Part model, mm, in its own coordinate system. Face numbers are marked on the shaded views. A direction names the side the tool comes from. Round coordinates to 2 decimals unless told otherwise and drop trailing zeros. Loops run counter-clockwise (first coordinate to the right, second up) from the corner with the lowest first, then second, coordinate; pieces in that order, holes last. Notation, with made-up numbers: (-3.75, 13.5) -> (38.25, 13.5) arc R21 cw to (38.25, 47.5) -> close; hole circle Ø2 at (55, 43). An arc over 180 degrees is marked (long way). Answer as CSV lines item,"result".
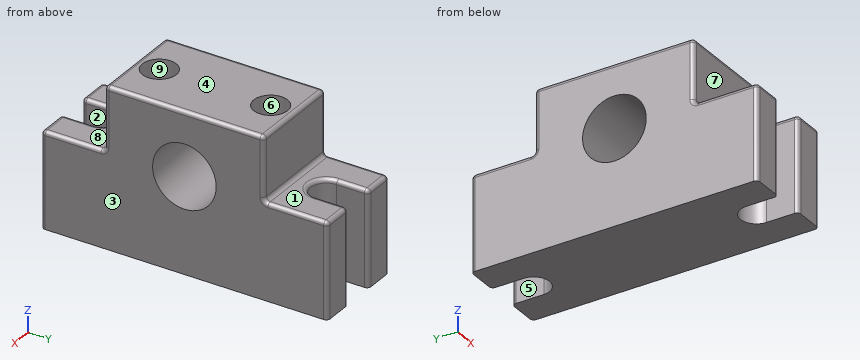
from build123d import *

# Parameters (mm, degrees)
F0_W     = 19.05
F0_H     = 6.35
F0_H_2   = 15.875
F0_R     = 3.571875
F0_H_3   = 9.525
F1_DEPTH = 19.05
F2_DEPTH = 31.75
F4_D     = 12.7
F6_D     = 6.7564
F6_DEPTH = 12.7
F6_TIP   = 2.0298273432
F7_R     = 0.79375


with BuildPart() as f1:
    # F0 (on Top) → F1 (new body)
    with BuildSketch(Plane.XY):
        with Locations((0, 3.175)):
            Rectangle(F0_W, F0_H)
        with BuildLine():
            Line((9.525, -28.575), (9.525, -15.875))
            Line((9.525, -15.875), (-9.525, -15.875))
            Line((-9.525, -15.875), (-9.525, -28.575))
            Line((-9.525, -28.575), (-3.175, -28.575))
            Line((-3.175, -28.575), (-3.175, -22.225))
            ThreePointArc((-3.175, -22.225), (0, -19.05), (3.175, -22.225))
            Line((3.175, -22.225), (3.175, -28.575))
            Line((3.175, -28.575), (9.525, -28.575))
        make_face()
        with Locations((0, -7.9375)):
            Rectangle(F0_W, F0_H_2)
        with Locations((0, -11.1125)):
            Circle(F0_R, mode=Mode.SUBTRACT)
        with Locations((0, 11.1125)):
            Rectangle(F0_W, F0_H_3)
        with Locations((0, 11.1125)):
            Circle(F0_R, mode=Mode.SUBTRACT)
        with BuildLine():
            Line((9.525, 15.875), (9.525, 28.575))
            Line((9.525, 28.575), (3.175, 28.575))
            Line((3.175, 28.575), (3.175, 22.225))
            ThreePointArc((3.175, 22.225), (0, 19.05), (-3.175, 22.225))
            Line((-3.175, 22.225), (-3.175, 28.575))
            Line((-3.175, 28.575), (-9.525, 28.575))
            Line((-9.525, 28.575), (-9.525, 15.875))
            Line((-9.525, 15.875), (9.525, 15.875))
        make_face()
        with Locations((0, 11.1125)):
            Circle(F0_R)
        with Locations((0, -11.1125)):
            Circle(F0_R)
    extrude(amount=F1_DEPTH)

    # F0 (on Top) → F2 (join)
    with BuildSketch(Plane.XY):
        with Locations((0, 3.175)):
            Rectangle(F0_W, F0_H)
        with Locations((0, -7.9375)):
            Rectangle(F0_W, F0_H_2)
        with Locations((0, -11.1125)):
            Circle(F0_R, mode=Mode.SUBTRACT)
        with Locations((0, 11.1125)):
            Rectangle(F0_W, F0_H_3)
        with Locations((0, 11.1125)):
            Circle(F0_R, mode=Mode.SUBTRACT)
        with Locations((0, -11.1125)):
            Circle(F0_R)
        with Locations((0, 11.1125)):
            Circle(F0_R)
    extrude(amount=F2_DEPTH)

    # F4 (through all)
    with Locations(Plane.YZ.offset(9.525)):
        with Locations((0, 19.05)):
            Hole(F4_D / 2)

    # F6
    with Locations(Plane.XY.offset(31.75)):
        with Locations((0, 11.1125), (0, -11.1125)):
            Hole(F6_D / 2, depth=F6_DEPTH)
            with Locations((0, 0, -(F6_DEPTH + F6_TIP / 2))):  # 118° drill point
                Cone(0, F6_D / 2, F6_TIP, mode=Mode.SUBTRACT)

    # F7
    f7_edges = [f1.edges().sort_by_distance(p)[0] for p in [
        (-9.525, 0, 31.75),
        (0, -15.875, 31.75),
        (9.525, 0, 31.75),
        (0, 15.875, 31.75),
        (9.525, 15.875, 25.4),
        (-9.525, 15.875, 25.4),
        (0, 15.875, 19.05),
        (9.525, 22.225, 19.05),
        (9.525, 28.575, 9.525),
        (-9.525, 28.575, 9.525),
        (6.35, 28.575, 19.05),
        (-6.35, 28.575, 19.05),
        (3.175, 28.575, 9.525),
        (-3.175, 28.575, 9.525),
        (3.175, 25.4, 19.05),
        (0, -15.875, 19.05),
        (9.525, -15.875, 25.4),
        (9.525, -22.225, 19.05),
        (-9.525, -22.225, 19.05),
        (-9.525, -15.875, 25.4),
        (-3.175, -25.4, 19.05),
        (6.35, -28.575, 19.05),
        (-6.35, -28.575, 19.05),
        (9.525, -28.575, 9.525),
        (-9.525, -28.575, 9.525),
        (3.175, -28.575, 9.525),
        (-3.175, -28.575, 9.525),
        (-9.525, 22.225, 19.05),
        (3.175, -25.4, 19.05),
        (0, -19.05, 19.05),
        (-3.175, 25.4, 19.05),
        (0, 19.05, 19.05),
    ]]
    fillet(f7_edges, radius=F7_R)


solid = f1.part
Q1. Saw through at B-B, the plane z = 22.5. Write the cut outline in (x, y) (1 decimal).
Geometry results:
outline,"(-9.5, -15.1) arc R0.8 ccw to (-8.7, -15.9) -> (8.7, -15.9) arc R0.8 ccw to (9.5, -15.1) -> (9.5, -5.3) -> (-9.5, -5.3) -> close; (-9.5, 5.3) -> (9.5, 5.3) -> (9.5, 15.1) arc R0.8 ccw to (8.7, 15.9) -> (-8.7, 15.9) arc R0.8 ccw to (-9.5, 15.1) -> close; hole circle Ø6.8 at (0, -11.1); hole circle Ø6.8 at (0, 11.1)"
Q2. Two-plate mould, pull along Y, no slides. Class the marked faces 6, 7, 8 and 9: pulls with the +Y half, pulls with the -Y half, needs draft (parallel to the pull), parting line crosses it, or undercut.
Geometry results:
face 6,"undercut"
face 7,"pulls with the -Y half"
face 8,"needs draft"
face 9,"undercut"
Q3. Drill centre lines: line 1 along Y through (x, z) = (-3, 24) (3 decimals); line 2 along Z through (x, y) = (-4, 0); line 3 along Y through (x, z) = (0, 23.5) (3 decimals). Where is each one in solid material? Low to high.
Geometry results:
line 1,"-15.875 to -12.666, -9.559 to -3.977, 3.977 to 9.559, 12.666 to 15.875"
line 2,"0 to 12.7, 25.4 to 31.75"
line 3,"-15.875 to -14.491, -7.734 to -4.53, 4.53 to 7.734, 14.491 to 15.875"
Q4. Drop flat-ended pins along their axis: P1, Ø2, axis at x = -3, z = 27, coming from the -Y side (3 decimals); P2, Ø7.5, axis at y = 0, z = 19.05, coming from the +X side; P3, Ø6, axis at x = 0, y = -11.11, coming from the +Z side; P4, Ø5.5, axis at x = -1, y = 21.5, coming from the +Z side. Give the stop position or say it passes through.
Geometry results:
P1,"y = -15.875"
P2,"through"
P3,"z = 18.82"
P4,"z = 19.05"
Q5. Which spindle directions (+Z, -Z, +X, -X, +Y, -Y) get a long thin tool onto all of the face, cutting with end or side? Do the marked faces 1, 2, 3, 4 and 5. Say none if no direction does.
Geometry results:
face 1,"+Z, +X, -X, +Y"
face 2,"+Z, -Z, -Y"
face 3,"+Z, -Z, +X, +Y, -Y"
face 4,"+Z, +X, -X, +Y, -Y"
face 5,"+Z, -Z, +Y"
